Design review of the part built by this model. Coordinates are the model's own, in mm. A direction names the side the tool comes from. Round coordinates to 2 decimals unless told otherwise and drop trailing zeros. Order: outer loops, then holes, each group sorted by start corner. A loop starts at its lowest first (then second) coordinate and runs counter-clockwise, first axis right, second up. Notation, with made-up numbers: (-6, 69) - (19, 69) arc R17 ccw to (19, 100) - close; hole circle Ø11 at (55, 44). An arc over 180 degrees is marked (long way). Use CSV: the item, a comma, the result in double quotes.
from build123d import *

# Parameters (mm, degrees)
SKETCH_1_W                  = 10
SKETCH_1_H                  = 20
SKETCH_1_W_2                = 8
SKETCH_1_H_2                = 25
EXTRUDE_1_DEPTH             = 10
HOLE_WIZARD_M4_1_AT_2_COUNT = 2
HOLE_WIZARD_M4_1_AT_2_PITCH = 34
HOLE_WIZARD_M4_1_2_D        = 4.5
HOLE_WIZARD_M4_1_2_DEPTH    = 10
SKETCH_7_R                  = 2.25
CUT_EXTRUDE_1_DEPTH         = 4


with BuildPart() as part:
    # 스케치1 → 보스-돌출1 (new body)
    with BuildSketch(Plane(origin=(0, 0, 0), x_dir=(1, 0, 0), z_dir=(0, 1, 0))):
        with Locations((0, 22.5)):
            Rectangle(SKETCH_1_W, SKETCH_1_H)
        Rectangle(SKETCH_1_W_2, SKETCH_1_H_2)
        with Locations((0, -22.5)):
            Rectangle(SKETCH_1_W, SKETCH_1_H)
    extrude(amount=EXTRUDE_1_DEPTH)

    # 스케치3 → Hole Wizard M4 _ _ _ _ _ _1 (revolve, cut)
    with BuildSketch(Plane(origin=(0, 10, -17), x_dir=(0, 0, 1), z_dir=(1, 0, 0))):
        Polygon((0, 0), (0, 10), (2.25, 10), (2.25, 4.4), (4, 4.4), (4, 0.7), (4.7, 0), align=None)
    hole_wizard_m4_1 = revolve(axis=Axis((0, 16.35, -17), (0, -1, 0)), mode=Mode.SUBTRACT)

    # Hole Wizard M4 _ _ _ _ _ _1 at 2: Hole Wizard M4 _ _ _ _ _ _1 ×2
    with Locations(*[(0, 0, i * HOLE_WIZARD_M4_1_AT_2_PITCH) for i in range(1, HOLE_WIZARD_M4_1_AT_2_COUNT)]):
        add(hole_wizard_m4_1, mode=Mode.SUBTRACT)

    # Hole Wizard M4 _ _1 2
    with Locations(Plane(origin=(0, 0, 0), x_dir=(-1, 0, 0), z_dir=(0, -1, 0))):
        with Locations((0, -27.5), (0, 27.5), (54.10839937, -109.42081154)):
            Hole(HOLE_WIZARD_M4_1_2_D / 2, depth=HOLE_WIZARD_M4_1_2_DEPTH)

    # 스케치7 → 컷-돌출1 (cut)
    with BuildSketch(Plane.XZ):
        Polygon((2.049593456, -31.05), (4.099186911, -27.5), (2.049593456, -23.95), (-2.049593456, -23.95), (-4.099186911, -27.5), (-2.049593456, -31.05), align=None)
        with Locations((0, -27.5)):
            Circle(SKETCH_7_R, mode=Mode.SUBTRACT)
        Polygon((2.049593456, 23.95), (-2.049593456, 23.95), (-4.099186911, 27.5), (-2.049593456, 31.05), (2.049593456, 31.05), (4.099186911, 27.5), align=None)
        with Locations((0, 27.5)):
            Circle(SKETCH_7_R, mode=Mode.SUBTRACT)
    extrude(amount=-CUT_EXTRUDE_1_DEPTH, mode=Mode.SUBTRACT)


solid = part.part
1) To check wall thickness, follow L1, parallel to Z at x = 0, y = 1.35; L2, parallel to Z at x = 0, y = 8.65; L3, parallel to X at y = 7.05, z = -17. State the ranges of each line that lie inside material, in increasing order. Write a range as from..to.
Data:
L1,"z = -32.5..-31.05, -23.95..-19.25, -14.75..14.75, 19.25..23.95, 31.05..32.5"
L2,"z = -32.5..-29.75, -25.25..-21, -13..13, 21..25.25, 29.75..32.5"
L3,"x = -5..-4, 4..5"
2) We need section A-A (y = 7.75). Give the boundary of the cut face in (x, z).
Data:
outline,"(-5, -32.5) - (5, -32.5) - (5, -12.5) - (4, -12.5) - (4, 12.5) - (5, 12.5) - (5, 32.5) - (-5, 32.5) - (-5, 12.5) - (-4, 12.5) - (-4, -12.5) - (-5, -12.5) - close; hole circle Ø8 at (0, -17); hole circle Ø8 at (0, 17); hole circle Ø4.5 at (0, -27.5); hole circle Ø4.5 at (0, 27.5)"
3) Insertion check: pin 1 Ø5 at (x, z) = (0, 17) entering from +Y; pin 2 Ø4 at (x, z) = (0, -17) entering from -Y; pin 3 Ø4 at (y, z) = (7, 9) entering from +X; pin 4 Ø1 at (y, z) = (2.5, -9) entering from -X. Each pin has a flat end and moves straight along its axis. Give the tip position at first contact, or say it passes through.
Data:
pin 1,"stops at y = 5.6"
pin 2,"passes through"
pin 3,"stops at x = 4"
pin 4,"stops at x = -4"
4) We need section C-C (y = 2.75). Give the boundary of the cut face in (x, z).
Data:
outline,"(-5, -32.5) - (5, -32.5) - (5, -12.5) - (4, -12.5) - (4, 12.5) - (5, 12.5) - (5, 32.5) - (-5, 32.5) - (-5, 12.5) - (-4, 12.5) - (-4, -12.5) - (-5, -12.5) - close; hole (-4.1, -27.5) - (-2.05, -31.05) - (2.05, -31.05) - (4.1, -27.5) - (2.05, -23.95) - (-2.05, -23.95) - close; hole (-4.1, 27.5) - (-2.05, 23.95) - (2.05, 23.95) - (4.1, 27.5) - (2.05, 31.05) - (-2.05, 31.05) - close; hole circle Ø4.5 at (0, -17); hole circle Ø4.5 at (0, 17)"
5) We need section B-B (z = -17). Give the boundary of the cut face in (x, y).
Data:
outline,"(-5, 0) - (-2.25, 0) - (-2.25, 5.6) - (-4, 5.6) - (-4, 9.3) - (-4.7, 10) - (-5, 10) - close; (2.25, 0) - (5, 0) - (5, 10) - (4.7, 10) - (4, 9.3) - (4, 5.6) - (2.25, 5.6) - close"
6) For faces 4 (the face through (0, 5, 32.5)), 5 (the face through (2, 5.6, -19)), 6 (the face through (3.06, 1.97, 29.3)), list the 3-axis set-ups (+Z, -Z, +X, -X, +Y, -Y) from which the entire face can be reached by the end or side of a thin tool; tool diameter is ignored.
Data:
face 4,"+Z, +X, -X, +Y, -Y"
face 5,"+Y"
face 6,"-Y"
7) The part is to be moulded in two halves that separate along X. For faces 1 (the face through (4.5, 4.9, -12.5)), 2 (the face through (0.86, 2.84, 19.08)), 3 (the face through (4, 5, 0)), say which applies: +X half, -X half, draft (parallel to the pull), parting line (faces both ways), or undercut.
Data:
face 1,"draft"
face 2,"undercut"
face 3,"+X half"
